Build history of the part. All positions in model axes, mm. Coordinates: 2 decimals unless noted, no trailing zeros. Order: outer loops, then holes, each group sorted by start corner. A loop starts at its lowest first (then second) coordinate and runs counter-clockwise, first axis right, second up. Notation, with made-up numbers: (40, 32.5) - (73, 32.5) arc R16 cw to (73, 41.5) - close; hole circle Ø3 at (75.25, 41). An arc over 180 degrees is marked (long way). Write each question's results on one line, items separated by ' | '.
from build123d import *

# Parameters (mm, degrees)
SHAPE_DEPTH        = 1000
CUT_EXTRUDE8_REACH = 20
SKETCH10_W         = 5.196152423
SKETCH10_H         = 136.851692929
SKETCH10_W_2       = 91.107695154
SKETCH10_W_3       = 23.696152423
SKETCH10_H_2       = 863.148307071


with BuildPart() as part:
    # Sketch1 → Shape (new body)
    with BuildSketch(Plane(origin=(0, 0, 0), x_dir=(1, 0, 0), z_dir=(0, 1, 0))):
        Polygon((-41.5, 0), (-60, 0), (-60, -9), (50.5, -9), (50.5, 0), (60, 0), (54.803847577, 9), (-36.303847577, 9), align=None)
    extrude(amount=SHAPE_DEPTH)

    # Sketch10 → Cut-Extrude8 (cut, up to next)
    with BuildSketch(Plane(origin=(0, 0, -9), x_dir=(-1, 0, 0), z_dir=(0, 0, -1)), mode=Mode.PRIVATE) as cut_extrude8_sk1:
        with Locations((-57.401923789, 931.574153536)):
            Rectangle(SKETCH10_W, SKETCH10_H)
    cut_extrude8_tool1 = extrude(cut_extrude8_sk1.sketch, amount=-CUT_EXTRUDE8_REACH, mode=Mode.PRIVATE) & part.part
    add(cut_extrude8_tool1.solids().sort_by_distance((57.401924, 931.574154, -9))[0], mode=Mode.SUBTRACT)
    # Sketch10 → Cut-Extrude8 (cut, up to next)
    with BuildSketch(Plane(origin=(0, 0, -9), x_dir=(-1, 0, 0), z_dir=(0, 0, -1)), mode=Mode.PRIVATE) as cut_extrude8_sk2:
        with Locations((-9.25, 931.574153536)):
            Rectangle(SKETCH10_W_2, SKETCH10_H)
    cut_extrude8_tool2 = extrude(cut_extrude8_sk2.sketch, amount=-CUT_EXTRUDE8_REACH, mode=Mode.PRIVATE) & part.part
    add(cut_extrude8_tool2.solids().sort_by_distance((9.25, 931.574154, -9))[0], mode=Mode.SUBTRACT)
    # Sketch10 → Cut-Extrude8 (cut, up to next)
    with BuildSketch(Plane(origin=(0, 0, -9), x_dir=(-1, 0, 0), z_dir=(0, 0, -1)), mode=Mode.PRIVATE) as cut_extrude8_sk3:
        with Locations((48.151923788, 931.574153536)):
            Rectangle(SKETCH10_W_3, SKETCH10_H)
    cut_extrude8_tool3 = extrude(cut_extrude8_sk3.sketch, amount=-CUT_EXTRUDE8_REACH, mode=Mode.PRIVATE) & part.part
    add(cut_extrude8_tool3.solids().sort_by_distance((-48.151924, 931.574154, -9))[0], mode=Mode.SUBTRACT)
    # Sketch10 → Cut-Extrude8 (cut, up to next)
    with BuildSketch(Plane(origin=(0, 0, -9), x_dir=(-1, 0, 0), z_dir=(0, 0, -1)), mode=Mode.PRIVATE) as cut_extrude8_sk4:
        with Locations((48.151923788, 431.574153536)):
            Rectangle(SKETCH10_W_3, SKETCH10_H_2)
    cut_extrude8_tool4 = extrude(cut_extrude8_sk4.sketch, amount=-CUT_EXTRUDE8_REACH, mode=Mode.PRIVATE) & part.part
    add(cut_extrude8_tool4.solids().sort_by_distance((-48.151924, 431.574154, -9))[0], mode=Mode.SUBTRACT)


solid = part.part
1. Drop flat-ended pins along their axis: pin 1 Ø3 at (y, z) = (426, -4.5) entering from +X; pin 2 Ø1.5 at (y, z) = (374.5, -2.5) entering from +X; pin 3 Ø1 at (y, z) = (520.5, -1.5) entering from +X; pin 4 Ø10.5 at (x, y) = (53, 491) entering from +Z. Give the stop position or say it passes through.
Solved:
pin 1: stops at x = 58.27 | pin 2: stops at x = 58.99 | pin 3: stops at x = 59.42 | pin 4: stops at z = 9
2. Band-saw the part on A-A on y = 729.5. Give the cut face in (x, z), then the cut area to 3 significant figures.
Solved:
outline: (-36.3, -9) - (54.8, -9) - (60, 0) - (50.5, 0) - (50.5, 9) - (-36.3, 9) - close | area: 1,620 mm2
3. Band-saw the part on B-B on z = 5.25. Give the cut face in (x, y), then the cut area to 3 significant figures.
Solved:
outline: (-36.3, 0) - (50.5, 0) - (50.5, 863.15) - (-36.3, 863.15) - close | area: 74,900 mm2
4. Probe line 1 (Z direction, x = 51, y = 749); line 2 (X direction, y = 50.5, z = 1); line 3 (X direction, y = 586.5, z = -0.25). List the from-to ranges inside material, lowest first.
Solved:
line 1: z = -9 to 0 | line 2: x = -36.3 to 50.5 | line 3: x = -36.3 to 59.86
